Geometry check sheet. Reference: the model listing, model coordinates, mm. Face numbers are marked on the shaded views. A direction names the side the tool comes from. Coordinates: 2 decimals unless noted, no trailing zeros. Write each loop counter-clockwise with the first axis right and the second up, starting at its lowest first coordinate (ties: lowest second). Pieces come first, ordered by that corner, then holes. Notation, with made-up numbers: M 55.5,47.25 L 84.5,47.25 A14 ccw 84.5,72.25 Z; hole C 44.25,14.25 d5. An arc over 180 degrees is marked long. Write each question's results on one line, items separated by ' | '.
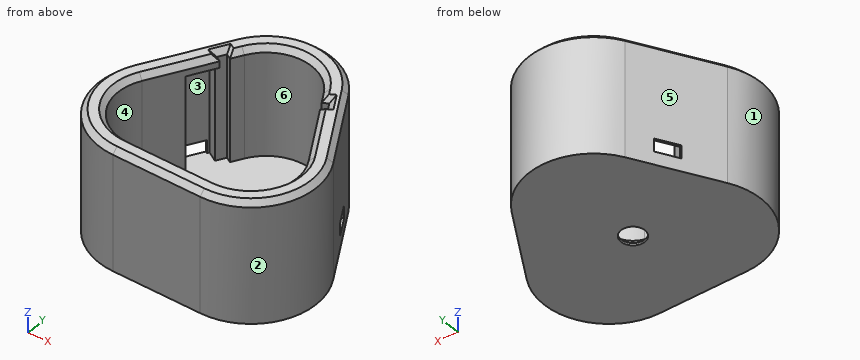
```python
from build123d import *

# Parameters (mm, degrees)
BOSS_EXTRU_1_DEPTH      = 25
ENL_V_MAT_EXTRU_1_DEPTH = 20
ENL_V_MAT_EXTRU_2_DEPTH = 45.21248121115924
ENL_V_MAT_EXTRU_4_DEPTH = 20
ENL_V_MAT_EXTRU_3_DEPTH = 45.21248121115924
CHANFREIN1_SIZE         = 1.2
BOSS_EXTRU_2_START      = 3
BOSS_EXTRU_2_DEPTH      = 3
ENL_V_MAT_EXTRU_5_REACH = 47.001
ESQUISSE7_W             = 1.399999999999995
ESQUISSE7_H             = 20
CHANFREIN2_SIZE2        = 4
CHANFREIN2_SIZE         = 2.309401077
ENL_V_MAT_EXTRU_6_REACH = 60.237
CHANFREIN3_SIZE2        = 4
CHANFREIN3_SIZE         = 2.309401077


with BuildPart() as part:
    # Esquisse1 → Boss.-Extru.1 (new body)
    with BuildSketch(Plane.XY):
        with BuildLine():
            Line((-22.99038105676658, 1.7264973081037391), (-12.990381056766578, 19.047005383792516))
            ThreePointArc((-12.990381056766578, 19.047005383792516), (9.5e-16, 26.547005383792516), (12.990381056766578, 19.047005383792513))
            Line((12.990381056766578, 19.047005383792513), (22.990381056766577, 1.726497308103746))
            ThreePointArc((22.990381056766577, 1.726497308103746), (22.99038105676658, -13.273502691896258), (9.999999999999996, -20.77350269189626))
            Line((9.999999999999996, -20.77350269189626), (-10, -20.773502691896258))
            ThreePointArc((-10, -20.773502691896258), (-22.99038105676658, -13.273502691896255), (-22.99038105676658, 1.7264973081037391))
        make_face()
        with BuildLine():
            Line((-18.66025403784439, -0.7735026918962613), (-8.66025403784439, 16.547005383792516))
            ThreePointArc((-8.66025403784439, 16.547005383792516), (-2.69e-15, 21.547005383792516), (8.660254037844384, 16.547005383792516))
            Line((8.660254037844384, 16.547005383792516), (18.660254037844386, -0.7735026918962474))
            ThreePointArc((18.660254037844386, -0.7735026918962474), (18.660254037844393, -10.773502691896258), (10, -15.773502691896258))
            Line((10, -15.773502691896258), (-10, -15.773502691896258))
            ThreePointArc((-10, -15.773502691896258), (-18.66025403784439, -10.773502691896262), (-18.66025403784439, -0.7735026918962613))
        make_face(mode=Mode.SUBTRACT)
    extrude(amount=BOSS_EXTRU_1_DEPTH)

    # Esquisse2 → Enlèv. mat.-Extru.1 (cut)
    with BuildSketch(Plane.XY.offset(25)):
        Polygon((-10.914359353944898, 12.642780450695335), (-12.300000000000002, 13.442780450695334), (-11.600000000000003, 14.655216015993549), (-10.2143593539449, 13.855216015993548), align=None)
        Polygon((10.214359353944896, 13.855216015993548), (11.6, 14.655216015993549), (12.299999999999999, 13.442780450695334), (10.914359353944896, 12.642780450695334), align=None)
    extrude(amount=-ENL_V_MAT_EXTRU_1_DEPTH, mode=Mode.SUBTRACT)

    # Esquisse3 → Enlèv. mat.-Extru.2 (cut, through all)
    with BuildSketch(Plane.XY.offset(25)):
        Polygon((-10.064359353944898, 14.115023637128878), (-11.709807621135333, 15.06502363712888), (-12.709807621135335, 13.332972829560003), (-11.064359353944898, 12.382972829560003), align=None)
    enl_v_mat_extru_2 = extrude(amount=-ENL_V_MAT_EXTRU_2_DEPTH, mode=Mode.SUBTRACT)

    # Symétrie1: Enlèv. mat.-Extru.2 across plane
    add(enl_v_mat_extru_2.mirror(Plane(origin=(0, 0, 0), x_dir=(0, 0, 1), z_dir=(1, 0, 0))), mode=Mode.SUBTRACT)

    # Esquisse6 → Enlèv. mat.-Extru.4 (cut)
    with BuildSketch(Plane(origin=(0, 0, 0), x_dir=(-1, 0, 0), z_dir=(0, 0, -1))):
        Polygon((11.250000000000002, 12.061433798642659), (15.147114317029969, 14.31143379864266), (18.297114317029976, 8.855473754800698), (14.4, 6.605473754800695), align=None)
        Polygon((-11.249999999999998, 12.061433798642659), (-15.14711431702997, 14.311433798642657), (-18.297114317029973, 8.855473754800693), (-14.399999999999997, 6.605473754800696), align=None)
    extrude(amount=-ENL_V_MAT_EXTRU_4_DEPTH, mode=Mode.SUBTRACT)

    # Esquisse5 → Enlèv. mat.-Extru.3 (cut, through all)
    with BuildSketch(Plane.XY.offset(25)):
        with BuildLine():
            Line((-9.093266739736611, 16.797005383792516), (-10.497372055837118, 14.365023637128878))
            Line((-10.497372055837118, 14.365023637128878), (-11.497372055837118, 12.632972829560003))
            Line((-11.497372055837118, 12.632972829560003), (-19.093266739736613, -0.5235026918962613))
            ThreePointArc((-19.093266739736613, -0.5235026918962613), (-19.09326673973661, -11.023502691896262), (-10.000000000000002, -16.273502691896258))
            Line((-10.000000000000002, -16.273502691896258), (10.000000000000004, -16.273502691896258))
            ThreePointArc((10.000000000000004, -16.273502691896258), (19.09326673973661, -11.023502691896251), (19.093266739736602, -0.523502691896249))
            Line((19.093266739736602, -0.523502691896249), (11.497372055837113, 12.632972829560005))
            Line((11.497372055837113, 12.632972829560005), (10.497372055837118, 14.36502363712888))
            Line((10.497372055837118, 14.36502363712888), (9.0932667397366, 16.797005383792516))
            ThreePointArc((9.0932667397366, 16.797005383792516), (-2.66e-15, 22.047005383792516), (-9.093266739736611, 16.797005383792516))
        make_face()
        with BuildLine():
            Line((-8.66025403784439, 16.547005383792516), (-10.064359353944898, 14.115023637128878))
            Line((-10.064359353944898, 14.115023637128878), (-11.064359353944894, 12.382972829560005))
            Line((-11.064359353944894, 12.382972829560005), (-18.66025403784439, -0.7735026918962613))
            ThreePointArc((-18.66025403784439, -0.7735026918962613), (-18.66025403784439, -10.773502691896262), (-10, -15.773502691896258))
            Line((-10, -15.773502691896258), (10.000000000000002, -15.77350269189626))
            ThreePointArc((10.000000000000002, -15.77350269189626), (18.66025403784439, -10.773502691896255), (18.660254037844386, -0.7735026918962474))
            Line((18.660254037844386, -0.7735026918962474), (11.064359353944898, 12.382972829560003))
            Line((11.064359353944898, 12.382972829560003), (10.064359353944898, 14.115023637128878))
            Line((10.064359353944898, 14.115023637128878), (8.660254037844384, 16.547005383792516))
            ThreePointArc((8.660254037844384, 16.547005383792516), (-2.69e-15, 21.547005383792516), (-8.66025403784439, 16.547005383792516))
        make_face(mode=Mode.SUBTRACT)
    extrude(amount=-ENL_V_MAT_EXTRU_3_DEPTH, mode=Mode.SUBTRACT)

    # Chanfrein1
    chanfrein1_edges = [part.edges().sort_by_distance(p)[0] for p in [
        (22.99038105676658, -13.27350269189626, 25),
        (11.103589838486222, 14.715023637128876, 25),
        (-11.103589838486226, 14.71502363712888, 25),
        (-9.795319397786868, 15.581014510460694, 25),
        (9.795319397786855, 15.581014510460696, 25),
        (-7.11e-15, 22.047005383792516, 25),
        (-15.295319397786866, 6.054735068831872, 25),
        (-19.09326673973661, -11.023502691896262, 25),
        (1.78e-15, -16.273502691896258, 25),
        (19.093266739736606, -11.023502691896253, 25),
        (15.295319397786855, 6.054735068831873, 25),
        (17.990381056766577, 10.386751345948129, 25),
        (2.66e-15, 26.547005383792516, 25),
        (-17.99038105676658, 10.386751345948127, 25),
        (-22.99038105676658, -13.273502691896258, 25),
        (-12.209807621135333, 14.19899823334444, 25),
        (-12.103589838486226, 12.982972829560003, 25),
        (-1.78e-15, -20.77350269189626, 25),
        (12.209807621135335, 14.19899823334444, 25),
        (12.103589838486222, 12.982972829560001, 25),
    ]]
    chamfer(chanfrein1_edges, length=CHANFREIN1_SIZE)

    # Esquisse4 → Boss.-Extru.2 (add)
    with BuildSketch(Plane(origin=(0, 0, 0), x_dir=(-1, 0, 0), z_dir=(0, 0, -1)).offset(BOSS_EXTRU_2_START)):
        with BuildLine():
            Line((22.99038105676658, 1.7264973081037323), (12.990381056766578, 19.047005383792516))
            ThreePointArc((12.990381056766578, 19.047005383792516), (8.9e-16, 26.547005383792513), (-12.990381056766573, 19.047005383792513))
            Line((-12.990381056766573, 19.047005383792513), (-22.990381056766577, 1.726497308103746))
            ThreePointArc((-22.990381056766577, 1.726497308103746), (-22.99038105676658, -13.273502691896255), (-10.000000000000004, -20.773502691896258))
            Line((-10.000000000000004, -20.773502691896258), (9.999999999999996, -20.773502691896258))
            ThreePointArc((9.999999999999996, -20.773502691896258), (22.990381056766577, -13.273502691896262), (22.99038105676658, 1.7264973081037323))
        make_face()
    extrude(amount=-BOSS_EXTRU_2_DEPTH)

    # Esquisse7 → Enlèv. mat.-Extru.5 (cut, up to next)
    with BuildSketch(Plane(origin=(-2.5958946838994956, 4.496221483611885, 0), x_dir=(0.866025403784439, 0.4999999999999994, 0), z_dir=(-0.4999999999999994, 0.866025403784439, 0)), mode=Mode.PRIVATE) as enl_v_mat_extru_5_sk1:
        with Locations((16.973502691896265, -10)):
            Rectangle(ESQUISSE7_W, ESQUISSE7_H)
    enl_v_mat_extru_5_tool1 = extrude(enl_v_mat_extru_5_sk1.sketch, amount=-ENL_V_MAT_EXTRU_5_REACH, mode=Mode.PRIVATE) & part.part
    enl_v_mat_extru_5 = enl_v_mat_extru_5_tool1.solids().sort_by_distance((12.10359, 12.982973, 10))[0]
    add(enl_v_mat_extru_5, mode=Mode.SUBTRACT)

    # Symétrie2: Enlèv. mat.-Extru.5 across plane
    add(enl_v_mat_extru_5.mirror(Plane(origin=(0, 0, 0), x_dir=(0, 0, 1), z_dir=(1, 0, 0))), mode=Mode.SUBTRACT)

    # Chanfrein2
    chanfrein2_edges = [part.edges().sort_by_distance(p)[0] for p in [
        (13.16519237886467, 9.74422329218035, 20),
    ]]
    chanfrein2_side = [part.faces().sort_by_distance(p)[0] for p in [
        (13.16519237886467, 9.74422329218035, 20.04618802153517),
    ]]
    chamfer(chanfrein2_edges, length=CHANFREIN2_SIZE - 0.0001, length2=CHANFREIN2_SIZE2 - 0.0001, reference=chanfrein2_side[0])  # a hair under: the kernel refuses the full size

    # Esquisse8 → Enlèv. mat.-Extru.6 (cut, up to next)
    with BuildSketch(Plane(origin=(17.557368354874363, 10.13675134594814, 0), x_dir=(0, 0, 1), z_dir=(-0.8660254037844385, -0.5000000000000004, 0)), mode=Mode.PRIVATE) as enl_v_mat_extru_6_sk1:
        Polygon((3.0000000000000004, 4.320508075688777), (5.3e-16, 4.320508075688777), (8.7e-16, -0.9794919243112247), (3.000000000000001, -0.9794919243112244), align=None)
    enl_v_mat_extru_6_tool1 = extrude(enl_v_mat_extru_6_sk1.sketch, amount=-ENL_V_MAT_EXTRU_6_REACH, mode=Mode.PRIVATE) & part.part
    enl_v_mat_extru_6 = enl_v_mat_extru_6_tool1.solids().sort_by_distance((16.722114, 11.583454, 1.5))[0]
    add(enl_v_mat_extru_6, mode=Mode.SUBTRACT)

    # Symétrie3: Enlèv. mat.-Extru.6 across plane
    add(enl_v_mat_extru_6.mirror(Plane(origin=(0, 0, 0), x_dir=(0, 0, 1), z_dir=(1, 0, 0))), mode=Mode.SUBTRACT)

    # Chanfrein3
    chanfrein3_edges = [part.edges().sort_by_distance(p)[0] for p in [
        (-13.16519237886467, 9.74422329218035, 20),
    ]]
    chanfrein3_side = [part.faces().sort_by_distance(p)[0] for p in [
        (-13.16519237886467, 9.74422329218035, 20.04618802153517),
    ]]
    chamfer(chanfrein3_edges, length=CHANFREIN3_SIZE - 0.0001, length2=CHANFREIN3_SIZE2 - 0.0001, reference=chanfrein3_side[0])  # a hair under: the kernel refuses the full size

    # Esquisse10 → Fraisage pour vis à tête fraisée M51 (revolve, cut)
    with BuildSketch(Plane(origin=(0, 0, 0), x_dir=(0, -1, 0), z_dir=(1, 0, 0))):
        Polygon((0, 0), (-7.3e-16, 2.9999999999999996), (2.7499999999999996, 2.9999999999999996), (2.75, 2.449999999999999), (5.200000000000001, 0), align=None)
    revolve(axis=Axis((0, 0, 6.349999999999991), (0, 0, -1)), mode=Mode.SUBTRACT)


solid = part.part
```
Q1. Scan lines: probe 1 along Y at (x, z) = (0, -2.55); probe 2 along X at (y, z) = (12.5, 9.5); probe 3 along Z at (x, y) = (-10, 5). Record each from-to range of solid material in increasing order.
Geometry check:
probe 1: y = -20.77 to -2.75, 2.75 to 26.55 | probe 2: x = -16.77 to -16.19, 16.19 to 16.77 | probe 3: z = -3 to 0
Q2. Sectioned sample at A-A on x = 0. Record the cut outline in (y, z).
Geometry check:
outline: M -20.77,-3 L -2.75,-3 L -2.75,-2.45 L -5.2,0 L -16.27,0 L -16.27,23.8 L -17.47,25 L -19.57,25 L -20.77,23.8 Z; M 2.75,-3 L 26.55,-3 L 26.55,23.8 L 25.35,25 L 23.25,25 L 22.05,23.8 L 22.05,0 L 5.2,0 L 2.75,-2.45 Z
Q3. Sectioned sample at B-B on z = 13.5. Record the cut outline in (x, y).
Geometry check:
outline: M -22.99,1.73 A15 ccw -10,-20.77 L 10,-20.77 A15 ccw 22.99,1.73 L 12.99,19.05 A15 ccw -12.99,19.05 Z; hole M -19.09,-0.52 A10.5 ccw -10,-16.27 L 10,-16.27 A10.5 ccw 19.09,-0.52 L 14.83,6.86 L 18.3,8.86 L 15.15,14.31 L 12.9,13.01 L 11.71,15.07 L 10.5,14.37 L 9.09,16.8 A10.5 ccw -9.09,16.8 L -10.5,14.37 L -11.71,15.07 L -12.9,13.01 L -15.15,14.31 L -18.3,8.86 L -14.83,6.86 Z
Q4. Access from +Z, -Z, +X, -X, +Y, -Y to the whole of each face (thin tool, end or side, straight path). Record for the marked faces 5 and 6.
Geometry check:
face 5: +Z, -Z, -X, +Y | face 6: +Z
Q5. Mould release check, pull along X, two halves, no side actions. Record for the marked faces 1, 2, 3 and 4: pulls with the +X half, pulls with the -X half, needs draft (parallel to the pull), parting line crosses it, or undercut.
Geometry check:
face 1: pulls with the -X half | face 2: pulls with the +X half | face 3: undercut | face 4: undercut
Q6. Depth check by flat-ended pin: P1, Ø6, axis at y = 2.5, z = 22, coming from the -X side; P2, Ø6, axis at y = 19.5, z = 20.5, coming from the +X side; P3, Ø10, axis at x = 1, z = 14.5, coming from the +Y side; P4, Ø5, axis at y = 14, z = 18, coming from the +X side. Enter the tip coordinate at first touch or a pass-through.
Geometry check:
P1: stops at x = -24.04 | P2: stops at x = 14.46 | P3: stops at y = 26.55 | P4: stops at x = 17.35
